from build123d import *

# Parameters (mm, degrees)
SKETCH1_R           = 14
BOSS_EXTRUDE1_DEPTH = 24
SKETCH2_R           = 1.5
CUT_EXTRUDE1_DEPTH  = 3
SKETCH3_R           = 4
BOSS_EXTRUDE2_DEPTH = 2


with BuildPart() as part:
    # Sketch1 → Boss-Extrude1 (new body)
    with BuildSketch(Plane(origin=(0, 0, 0), x_dir=(1, 0, 0), z_dir=(0, 1, 0))):
        Circle(SKETCH1_R)
    extrude(amount=BOSS_EXTRUDE1_DEPTH)

    # Sketch2 → Cut-Extrude1 (cut)
    with BuildSketch(Plane(origin=(0, 24, 0), x_dir=(1, 0, 0), z_dir=(0, 1, 0))):
        with Locations((8, 0)):
            Circle(SKETCH2_R)
        with Locations((0, 9.5)):
            Circle(SKETCH2_R)
        with Locations((-8, 0)):
            Circle(SKETCH2_R)
        with Locations((0, -9.5)):
            Circle(SKETCH2_R)
    extrude(amount=-CUT_EXTRUDE1_DEPTH, mode=Mode.SUBTRACT)

    # Sketch3 → Boss-Extrude2 (add)
    with BuildSketch(Plane.XZ):
        Circle(SKETCH3_R)
    extrude(amount=BOSS_EXTRUDE2_DEPTH)


solid = part.part
Geometry check sheet. Reference: the model listing, model coordinates, mm. A direction names the side the tool comes from. Give positions to 0.01 mm unless a question says otherwise; leave off trailing zeros. Order: outer loops, then holes, each group sorted by start corner. A loop starts at its lowest first (then second) coordinate and runs counter-clockwise, first axis right, second up. Notation, with made-up numbers: (10, 65) - (41, 65) arc R21 cw to (41, 97) - close; hole circle Ø8 at (19, 54). An arc over 180 degrees is marked (long way). Use one line per item in the form item = value.
1) Sectioned sample at D-D (z = -9.5). Record the boundary of the cut face in (x, y), and give its area (3 significant figures).
Working result:
outline = (-10.28, 0) - (10.28, 0) - (10.28, 24) - (1.5, 24) - (1.5, 21) - (-1.5, 21) - (-1.5, 24) - (-10.28, 24) - close
area = 485 mm^2
2) Sectioned sample at B-B (x = 0). Record the boundary of the cut face in (y, z).
Working result:
outline = (-2, -4) - (0, -4) - (0, -14) - (24, -14) - (24, -11) - (21, -11) - (21, -8) - (24, -8) - (24, 8) - (21, 8) - (21, 11) - (24, 11) - (24, 14) - (0, 14) - (0, 4) - (-2, 4) - close
3) Depth check by flat-ended pin: pin 1 Ø1 at (x, y) = (-9.5, 11) entering from +Z; pin 2 Ø2 at (x, y) = (11, 13) entering from +Z; pin 3 Ø1 at (y, z) = (19.5, -1) entering from +X. Enter the tip coordinate at first touch or a pass-through.
Working result:
pin_1 = 10.72
pin_2 = 9.8
pin_3 = 13.99
4) Draft check along X on faces 4 (the face through (12.932, 11.832, 5.362)), 5 (the face through (0, 23, 11)), 6 (the face through (0, 23, -8)), 7 (the face through (0, -2, 0)). Enter one of: released by +X, released by -X, zero draft, split by the parting line, or undercut.
Working result:
face_4 = split by the parting line
face_5 = undercut
face_6 = undercut
face_7 = zero draft
5) Access from +Z, -Z, +X, -X, +Y, -Y to the whole of each face (thin tool, end or side, straight path). Record for faces 1 (the face through (0, 24, 0)), 2 (the face through (-0.867, -0.986, -3.905)), 3 (the face through (8, 21, 0)).
Working result:
face_1 = +Z, -Z, +X, -X, +Y
face_2 = -Y
face_3 = +Y
6) Material ranges on probe 1 along Z at (x, y) = (0, 22.7); probe 2 along X at (y, z) = (22.95, 0); probe 3 along Y at (x, z) = (-11, -7.25), recorded low to high. Write a range as from..to.
Working result:
probe_1 = -14..-11, -8..8, 11..14
probe_2 = -14..-9.5, -6.5..6.5, 9.5..14
probe_3 = 0..24
7) Sectioned sample at C-C (y = 4). Record the boundary of the cut face in (x, z).
Working result:
outline = circle Ø28 at (0, 0)
8) Sectioned sample at A-A (z = 0). Record the boundary of the cut face in (x, y).
Working result:
outline = (-14, 0) - (-4, 0) - (-4, -2) - (4, -2) - (4, 0) - (14, 0) - (14, 24) - (9.5, 24) - (9.5, 21) - (6.5, 21) - (6.5, 24) - (-6.5, 24) - (-6.5, 21) - (-9.5, 21) - (-9.5, 24) - (-14, 24) - close
